For this review, take the finished solid that the model builds, in its own axes (mm). Round coordinates to 2 decimals unless told otherwise and drop trailing zeros. Loops run counter-clockwise (first coordinate to the right, second up) from the corner with the lowest first, then second, coordinate; pieces in that order, holes last. Notation, with made-up numbers: (-35, 25) -> (-15, 25) arc R10 ccw to (-15, 33) -> close; hole circle Ø11 at (9.25, -22). An arc over 180 degrees is marked (long way). Write each question's results on one line, items separated by ' | '.
```python
from build123d import *

# Parameters (mm, degrees)
ESQUISSE1_R        = 10
BOSS_EXTRU_1_DEPTH = 5


with BuildPart() as part:
    # Esquisse1 → Boss.-Extru.1 (new, symmetric)
    with BuildSketch(Plane.XY):
        with BuildLine():
            Line((0, -15), (-200, -15))
            ThreePointArc((-200, -15), (-215, 0), (-200, 15))
            Line((-200, 15), (0, 15))
            ThreePointArc((0, 15), (15, 0), (0, -15))
        make_face()
        with Locations((-200, 0)):
            Circle(ESQUISSE1_R, mode=Mode.SUBTRACT)
        Circle(ESQUISSE1_R, mode=Mode.SUBTRACT)
    extrude(amount=BOSS_EXTRU_1_DEPTH, both=True)


solid = part.part
```
1. Draft analysis for pull direction X (two halves, no side actions). For faces 1 (the face through (-2.17, -9.76, -0.07)), 2 (the face through (15, 0, 0)), 3 (the face through (-99, -15, 0)), state which applies: released by +X, released by -X, zero draft, split by the parting line, or undercut.
Values found:
face 1: undercut | face 2: released by +X | face 3: zero draft
2. Consider section A-A (y = 0). State the section outline as (x, z) points, plus the area to 3 significant figures.
Values found:
outline: (-215, -5) -> (-210, -5) -> (-210, 5) -> (-215, 5) -> close; (-190, -5) -> (-10, -5) -> (-10, 5) -> (-190, 5) -> close; (10, -5) -> (15, -5) -> (15, 5) -> (10, 5) -> close | area: 1,900 mm2
3. Consider section B-B (z = -3.25). State the section outline as (x, y) points.
Values found:
outline: (-200, -15) -> (0, -15) arc R15 ccw to (0, 15) -> (-200, 15) arc R15 ccw to start; hole circle Ø20 at (-200, 0); hole circle Ø20 at (0, 0)
4. To check wall thickness, follow probe 1 along X at (y, z) = (-0.5, -0.5); probe 2 along Y at (x, z) = (-200, -1.5); probe 3 along X at (y, z) = (-8, 1.5). State the ranges of each line that lie inside material, in increasing order.
Values found:
probe 1: x = -214.99 to -209.99, -190.01 to -9.99, 9.99 to 14.99 | probe 2: y = -15 to -10, 10 to 15 | probe 3: x = -212.69 to -206, -194 to -6, 6 to 12.69
5. Consider section C-C (y = 13). State the section outline as (x, z) points.
Values found:
outline: (-207.48, -5) -> (7.48, -5) -> (7.48, 5) -> (-207.48, 5) -> close
6. For pin 1 (3 mm diameter, centred on y = -3, z = 0, fed in from +X); pin 2 (6 mm diameter, centred on y = 3.5, z = -1.5, fed in from +X); pin 3 (4 mm diameter, centred on y = 9.5, z = -1, fed in from +X), all flat-tipped, find the tip position at first contact; note any pin that passes through.
Values found:
pin 1: stops at x = 14.92 | pin 2: stops at x = 14.99 | pin 3: stops at x = 12.99
